Check sheet for the modelled part. Datum: model origin and axes. Units: mm. Coordinates: 2 decimals unless noted, no trailing zeros. Order: outer loops, then holes, each group sorted by start corner. A loop starts at its lowest first (then second) coordinate and runs counter-clockwise, first axis right, second up.
1. Cross-section at B-B (x = 225.05). Count the separate pieces of the cut face and the enclosed holes in it, then the cut area to 3 significant figures.
2. Thickness scan on line 1 (Y direction, x = 222.9, z = 40); line 2 (Z direction, x = 223.35, y = 15); line 3 (Y direction, x = 223.05, z = -25.5). Record the ranges inside material, lowest first.
3. Cross-section at A-A (z = 43). Enter the section's corners in (x, y).
4. Gauge pin test, flat end, axial feed: pin 1 Ø1 at (y, z) = (17.5, 37) entering from +X. Record the tip position at first contact, or that the pin passes through.
Autodesk Inventor part; units mm, degrees
ref_plane "YZ Plane" through (0, 0, 0) normal (1, 0, 0) x (0, 1, 0)
ref_plane "XZ Plane" through (0, 0, 0) normal (0, 1, 0) x (-1, 0, 0)
ref_plane "XY Plane" through (0, 0, 0) normal (0, 0, 1) x (1, 0, 0)
sketch "Sketch1" plane through (0, 0, 0) normal (0, 0, 1) x (1, 0, 0)
  arc A0 (180.1312, 23.4516) -> (181.5833, 23.6751) centre (180.1312, 28.2803) ccw
  arc A1 (180.1312, 23.4516) -> (181.5842, 23.6753) centre (180.1312, 28.2803) ccw
  arc A2 (180.1312, 21.4516) -> (182.1847, 21.7676) centre (180.1312, 28.2803) ccw
  arc A3 (167.724, 26.7761) -> (180.1312, 23.4516) centre (180.1312, 48.266) ccw
  arc A4 (166.724, 25.044) -> (180.1312, 21.4516) centre (180.1312, 48.266) ccw
  arc A5 (166.724, 53.0576) -> (167.724, 52.0576) centre (167.724, 53.0576) ccw
  line L0 (233.0254, 52.0576) -> (167.724, 52.0576)
  line L1 (233.0254, 54.0576) -> (169.724, 54.0576)
  line L2 (182.1847, 21.7676) -> (237.115, 39.0871)
  line L3 (236.5136, 40.9945) -> (181.5833, 23.6751)
  line L4 (168.724, 25.044) -> (168.724, 31.7835)
  line L5 (166.724, 25.044) -> (166.724, -4.6444)
  line L6 (236.5136, 40.9945) -> (237.115, 39.0871)
  line L7 (233.0254, 52.0576) -> (237.115, 52.0576)
  line L8 (233.0254, 54.0576) -> (237.115, 54.0576)
  line L9 (237.115, 52.0576) -> (237.115, 54.0576)
  line L10 (0, 3.5755) -> (319.1694, 3.5755)
  line L11 (0, 88.1805) -> (30.0219, 88.1805)
  line L12 (30.0219, 90.1805) -> (0, 90.1805)
  line L13 (0, 88.1805) -> (0, 90.1805)
  line L14 (0, 77.0805) -> (30.0219, 77.0805)
  line L15 (0, 75.0805) -> (30.0219, 75.0805)
  line L16 (124.3912, 51.7943) -> (167.724, 26.7761)
  line L17 (123.3912, 50.0622) -> (166.724, 25.044)
  line L18 (166.724, 25.044) -> (166.724, 31.1529)
  arc A6 (123.3912, 50.0622) -> (30.0219, 75.0805) centre (30.0219, -111.6581) ccw
  arc A7 (124.3912, 51.7943) -> (30.0219, 77.0805) centre (30.0219, -111.6581) ccw
  line L19 (30.0219, 88.1805) -> (165.724, 88.1805)
  line L20 (167.724, 90.1805) -> (30.0219, 90.1805)
  line L21 (166.724, 53.0576) -> (166.724, 87.1805)
  line L22 (168.724, 55.0576) -> (168.724, 89.1805)
  arc A8 (168.724, 55.0576) -> (169.724, 54.0576) centre (169.724, 55.0576) ccw
  arc A9 (166.724, 87.1805) -> (165.724, 88.1805) centre (165.724, 87.1805) ccw
  arc A10 (168.724, 89.1805) -> (167.724, 90.1805) centre (167.724, 89.1805) ccw
  line L23 (236.5136, 40.9945) -> (236.5136, 52.0576)
  line L24 (236.5136, 52.0576) -> (233.5136, 52.0576)
  line L25 (233.5136, 52.0576) -> (233.5136, 40.0486)
  line L26 (233.5136, 52.0576) -> (225.5136, 52.0576)
  line L27 (225.5136, 52.0576) -> (225.5136, 37.5262)
  line L28 (225.5136, 52.0576) -> (222.5136, 52.0576)
  line L29 (222.5136, 52.0576) -> (222.5136, 36.5803)
  line L30 (233.0254, 52.0576) -> (225.5136, 49.6892)
  line L31 (222.5136, 48.7433) -> (144.4694, 24.136)
  dimension "d18" = 30.0219
  dimension "d19" = 186.7386
  dimension "d20" = 0
  dimension "d21" = 0
  dimension "d22" = 71.505
  dimension "d23" = 2
  dimension "d24" = 2
  dimension "d25" = 2
  dimension "d26" = 2
  dimension "d27" = 2
  dimension "d28" = 17.5
  dimension "d29" = 54.9303
  dimension "d30" = 2
  dimension "d31" = 11.1
  dimension "d32" = 11.6
  dimension "d34" = 2
  dimension "d35" = 2
  dimension "d36" = 1
  dimension "d37" = 1
  dimension "d38" = 1
  dimension "d39" = 1
  dimension "d40" = 3
  dimension "d41" = 8
  dimension "d42" = 3
revolve "Revolution1" add sketch "Sketch1" angle 360 about axis through (0, 3.5755, 0) along (1, 0, 0) contours L29 L0 L27 L3
sketch "Sketch4" plane through (225.5136, 3.5755, 0) normal (1, 0, 0) x (0, 0, -1)
  circle A0 centre (0, 0) radius 33.9508
  line L0 (0, 33.9508) -> (0, 38.7133)
  circle A1 centre (0, 38.7133) radius 4.7625
  point P0 (0, -3.5755)
  dimension "d47" = 4.7625
  dimension "d48" = 9.525
sketch "Sketch5" plane through (222.5136, 3.5755, 0) normal (-1, 0, 0) x (0, 0, 1)
  circle A0 centre (0, 0) radius 33.0049
  line L0 (0, 33.0049) -> (0, 37.7674)
  circle A1 centre (0, 37.7674) radius 4.7625
  point P0 (0, -3.5755)
  dimension "d49" = 4.7625
  dimension "d50" = 9.525
sketch "Sketch6" plane through (0, 0, 0) normal (0, 0, 1) x (1, 0, 0)
  line L0 (225.5136, -44.9067) -> (225.5136, 52.0576)
  line L1 (225.5136, 42.2627) -> (222.5136, 41.3779)
  line L2 (222.5136, -44.9067) -> (222.5136, 52.0576)
  point P0 (0, 0)
sweep "Sweep1" cut profiles "Sketch4" path "Sketch6" path curves L1 contours A1
pattern_circular "Circular Pattern1" count 10 over 360 about axis through (224.0136, 3.5755, 0) along (1, 0, 0) of "Sweep1"
sketch "Sketch7" plane through (225.5136, 3.5755, 0) normal (1, 0, 0) x (0, 0, -1)
  circle A0 centre (0, 0) radius 48.4822
  line L0 (0, 48.4822) -> (0, 47.9822)
  line L1 (0.25, 47.7322) -> (-0.25, 47.7322)
  line L2 (-0.25, 47.7322) -> (-0.25, 48.2322)
  line L3 (-0.25, 48.2322) -> (0.25, 48.2322)
  line L4 (0.25, 48.2322) -> (0.25, 47.7322)
  line L5 (0.25, 47.7322) -> (-0.25, 48.2322) construction
  line L6 (-0.25, 47.7322) -> (0.25, 48.2322) construction
  point P0 (0, -3.5755)
  dimension "d56" = 0.5
  dimension "d60" = 0.5
  dimension "d61" = 0.5
extrude "Extrusion1" cut sketch "Sketch7" against normal blind 10 contours L1 L2 L3 L4
properties part number "back bracket 2" material "Stainless Steel"
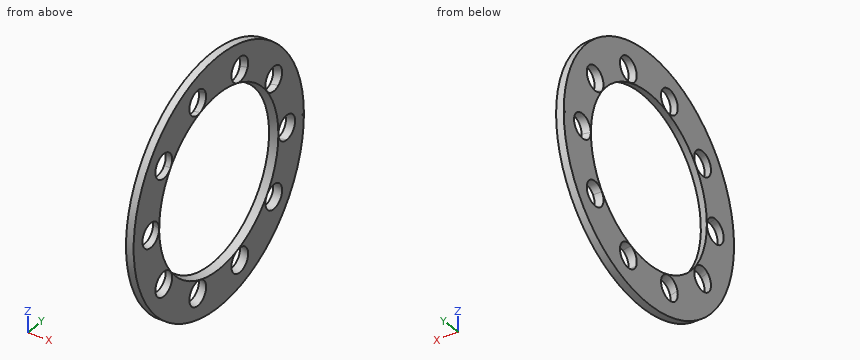
Data:
1. separate pieces: 1
1. enclosed holes: 12
1. area: 3,080 mm2
2. line 1: y = -23.82 to -10.86, -5.44 to 12.59, 18.01 to 30.97
2. line 2: z = -47.12 to -40.96, -31.46 to -31.25, 31.25 to 31.46, 40.96 to 47.12
2. line 3: y = -37.66 to -30.71, -23.6 to -17.64, 24.79 to 30.75, 37.86 to 44.81
3. outline: (222.51, -18.82) - (225.51, -18.82) - (225.51, 25.97) - (222.51, 25.97) - close
4. pin 1: passes through
